Geometry: final body of the model. Coordinates: model frame, mm. Face numbers are marked on the shaded views. Round coordinates to 2 decimals unless told otherwise and drop trailing zeros. Loops run counter-clockwise (first coordinate to the right, second up) from the corner with the lowest first, then second, coordinate; pieces in that order, holes last. Notation, with made-up numbers: M 53.5,62.5 L 57.5,62.5 A30 ccw 57.5,97.5 Z; hole C 89.5,15 d7. An arc over 180 degrees is marked long. Write each question's results on one line, items separated by ' | '.
Autodesk Inventor part; units mm, degrees
ref_plane "Work Plane4" through (0, 17.5, 0) normal (0, 1, 0) x (-1, 0, 0)
ref_plane "Work Plane3" through (0, 17.5, 0) normal (0, 1, 0) x (-1, 0, 0)
ref_plane "Work Plane5" through (0, 13.96, 0) normal (0, 1, 0) x (-1, 0, 0)
sketch "Sketch3" plane through (0, 0, 0) normal (0, 0, 1) x (1, 0, 0)
  circle A0 centre (0, 0) radius 17.25
  circle A1 centre (0, 0) radius 17.375
  dimension "d8" = 34.5
  dimension "d9" = 34.75
extrude "Extrusion3" add sketch "Sketch3" along normal mid plane 6.25
sketch "Sketch4" plane through (0, 0, 3.125) normal (0, 0, 1) x (1, 0, 0)
  circle A0 centre (0, 0) radius 17.375
  circle A1 centre (0, 0) radius 17.625
  dimension "d12" = 34.75
  dimension "d13" = 0.25
extrude "Extrusion4" cut sketch "Sketch4" along normal blind 0.25 and the other way blind 5.75
ref_plane "Work Plane4" through (0, 17.5, 0) normal (0, 1, 0) x (-1, 0, 0)
sketch "Sketch6" plane through (0, 17.5, 0) normal (0, 1, 0) x (-1, 0, 0)
  line L0 (-10, 3.75) -> (10, 3.75)
  line L1 (10, 3.75) -> (10, -3.75)
  line L2 (10, -3.75) -> (-10, -3.75)
  line L3 (-10, -3.75) -> (-10, 3.75)
  line L4 (-10, 3.75) -> (10, -3.75) construction
  line L5 (10, 3.75) -> (-10, -3.75) construction
  point P0 (0, 0)
  dimension "d19" = 20
  dimension "d20" = 7.5
extrude "Extrusion5" cut sketch "Sketch6" against normal blind 10
ref_plane "Work Plane3" through (0, 17.5, 0) normal (0, 1, 0) x (-1, 0, 0)
sketch "Sketch7" plane through (0, 17.5, 0) normal (0, 1, 0) x (-1, 0, 0)
  point P0 (0, 0)
sketch "Sketch8" plane through (10, 14.0557, -3.125) normal (-1, 0, 0) x (0, 0, 1)
  line L0 (6.25, 0) -> (0, 0)
  line L1 (0, 0) -> (0, 0.1531)
  line L2 (0, 0.1531) -> (6.25, 0.1531)
  line L3 (6.25, 0.1531) -> (0, 0.1531)
  point P0 (3.125, 0.1531)
  point P1 (3.125, 0.1531)
ref_plane "Work Plane5" through (0, 13.96, 0) normal (0, 1, 0) x (-1, 0, 0)
sketch "Sketch9" plane through (0, 13.96, 0) normal (0, 1, 0) x (-1, 0, 0)
  line L0 (-10, -3.125) -> (-10, 3.125)
  line L1 (10, -3.125) -> (-10, -3.125)
  line L2 (-10, -3.125) -> (-10, 3.125)
  line L3 (-10, 3.125) -> (10, 3.125)
  line L4 (10, 3.125) -> (10, -3.125)
  point P0 (0, 0)
extrude "Extrusion6" add sketch "Sketch9" along normal blind 0.25
properties part number "Small_Ring" material "Iron, Cast"
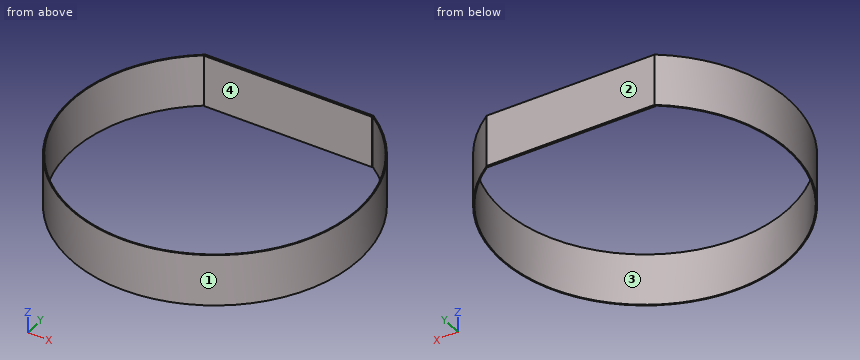
1. Section C-C (y = 0). Output: boundary loops of the cut face in (x, z) (3 decimals).
Answer key:
outline: M -17.375,-3.125 L -17.25,-3.125 L -17.25,3.125 L -17.375,3.125 Z; M 17.25,-3.125 L 17.375,-3.125 L 17.375,3.125 L 17.25,3.125 Z
2. Ray query, probe 1 along Y at (x, z) = (13, -2.25); probe 2 along Y at (x, z) = (-14, 2); probe 3 along X at (y, z) = (-11, 1.25). Return the intervals inside material, ascending.
Answer key:
probe 1: y = -11.53 to -11.34, 11.34 to 11.53 | probe 2: y = -10.29 to -10.08, 10.08 to 10.29 | probe 3: x = -13.45 to -13.29, 13.29 to 13.45
3. Section A-A (x = 0). Output: boundary loops of the cut face in (y, z) (3 decimals), then the cut area to 3 significant figures.
Answer key:
outline: M -17.375,-3.125 L -17.25,-3.125 L -17.25,3.125 L -17.375,3.125 Z; M 13.96,-3.125 L 14.21,-3.125 L 14.21,3.125 L 13.96,3.125 Z | area: 2.34 mm²
4. Pin query (flat end, axial travel): P1, Ø1.5, axis at y = -6, z = -0.5, coming from the +X side; P2, Ø1, axis at x = 7.5, z = 1, coming from the -Y side; P3, Ø2, axis at y = 1.5, z = 1.5, coming from the +X side. Return the tip coordinate at first contact, or that it passes through.
Answer key:
P1: stops at x = 16.56 | P2: stops at y = -15.9 | P3: stops at x = 17.37
5. Draft query along Y for the marked faces 1, 2, 3 and 4. Return one class per face: pulls with the +Y half, pulls with the -Y half, needs draft (parallel to the pull), parting line crosses it, or undercut.
Answer key:
face 1: parting line crosses it | face 2: pulls with the +Y half | face 3: undercut | face 4: undercut
